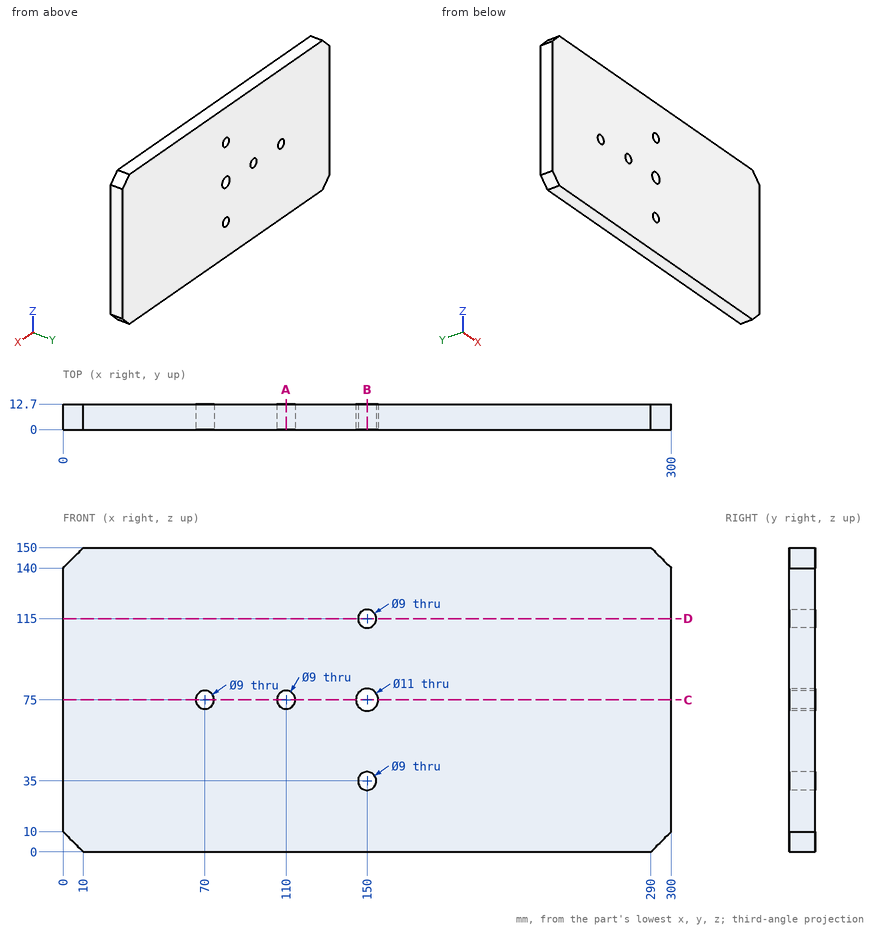
The drawing under review shows one solid part. Ordinate dimensions are in mm from its lowest x, y, z. Give positions to 0.01 mm unless a question says otherwise; leave off trailing zeros. Write each loop counter-clockwise with the first axis right and the second up, starting at its lowest first coordinate (ties: lowest second). Pieces come first, ordered by that corner, then holes. Notation, with made-up numbers: (49, 56) - (54, 56) arc R5 ccw to (54, 62) - close; hole circle Ø5 at (73.25, -39.5). An arc over 180 degrees is marked (long way). Answer in a Markdown table with one row per item. Add a question column.
1. Wall thickness on line 1 along X through (y, z) = (7.25, 75); line 2 along Z through (x, y) = (150, 5.5); line 3 along X through (y, z) = (4.25, 35): over which ranges is each line inside the solid? List them lowest first. Write a range as [from, to].
2. We need section C-C on z = 75. Write out the cut boundary in (x, y).
3. We need section A-A on x = 110. Write out the cut boundary in (y, z).
4. We need section D-D on z = 115. Write out the cut boundary in (x, y).
5. We need section B-B on x = 150. Write out the cut boundary in (y, z), then the cut area to 3 significant figures.
Ans:
| question | item | result |
|---|---|---|
| 1 | line 1 | x = [0, 65.5], [74.5, 105.5], [114.5, 144.5], [155.5, 300] |
| 1 | line 2 | z = [0, 30.5], [39.5, 69.5], [80.5, 110.5], [119.5, 150] |
| 1 | line 3 | x = [0, 145.5], [154.5, 300] |
| 2 | outline | (0, 0) - (65.5, 0) - (65.5, 12.7) - (0, 12.7) - close; (74.5, 0) - (105.5, 0) - (105.5, 12.7) - (74.5, 12.7) - close; (114.5, 0) - (144.5, 0) - (144.5, 12.7) - (114.5, 12.7) - close; (155.5, 0) - (300, 0) - (300, 12.7) - (155.5, 12.7) - close |
| 3 | outline | (0, 0) - (12.7, 0) - (12.7, 70.5) - (0, 70.5) - close; (0, 79.5) - (12.7, 79.5) - (12.7, 150) - (0, 150) - close |
| 4 | outline | (0, 0) - (145.5, 0) - (145.5, 12.7) - (0, 12.7) - close; (154.5, 0) - (300, 0) - (300, 12.7) - (154.5, 12.7) - close |
| 5 | outline | (0, 0) - (12.7, 0) - (12.7, 30.5) - (0, 30.5) - close; (0, 39.5) - (12.7, 39.5) - (12.7, 69.5) - (0, 69.5) - close; (0, 80.5) - (12.7, 80.5) - (12.7, 110.5) - (0, 110.5) - close; (0, 119.5) - (12.7, 119.5) - (12.7, 150) - (0, 150) - close |
| 5 | area | 1,540 mm^2 |
